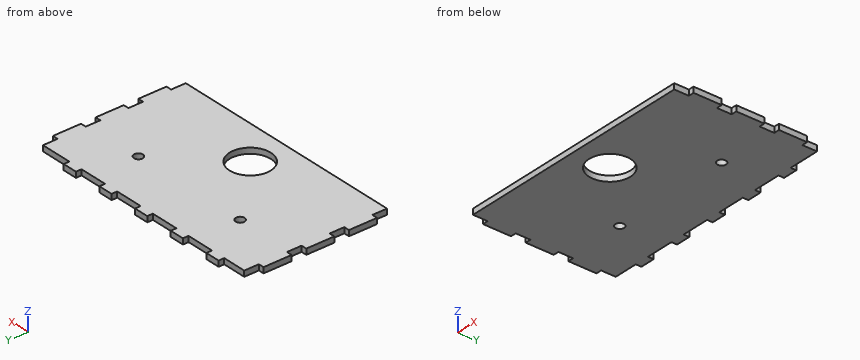
from build123d import *

# Parameters (mm, degrees)
SKETCH1_W               = 134.64
SKETCH1_H               = 76.2
BOSS_EXTRUDE1_DEPTH     = 3
SKETCH2_W               = 3
SKETCH2_H               = 7.8
CUT_EXTRUDE1_DEPTH      = 78.411836304
LPATTERN1_COUNT         = 4
LPATTERN1_PITCH         = 22.8
MIRROR4_COPY_1_SKETCH_W = 3
MIRROR4_COPY_1_SKETCH_H = 7.8
MIRROR4_COPY_1_DEPTH    = 78.411836304
MIRROR4_COPY_2_SKETCH_W = 3
MIRROR4_COPY_2_SKETCH_H = 7.8
MIRROR4_COPY_2_DEPTH    = 78.411836304
MIRROR4_COPY_3_SKETCH_W = 3
MIRROR4_COPY_3_SKETCH_H = 7.8
MIRROR4_COPY_3_DEPTH    = 78.411836304
SKETCH3_W               = 7.8
SKETCH3_H               = 3
BOSS_EXTRUDE2_DEPTH     = 3
LPATTERN2_COUNT         = 5
LPATTERN2_PITCH         = 22.8
SKETCH4_R               = 11
CUT_EXTRUDE2_DEPTH      = 79.931567829
SKETCH5_R               = 2.3749
CUT_EXTRUDE3_DEPTH      = 79.931567829


with BuildPart() as part:
    # Sketch1 → Boss-Extrude1 (new body)
    with BuildSketch(Plane.XY):
        Rectangle(SKETCH1_W, SKETCH1_H)
    extrude(amount=BOSS_EXTRUDE1_DEPTH)

    # Sketch2 → Cut-Extrude1 (cut, through all)
    with BuildSketch(Plane.XY.offset(3)):
        with Locations((-65.82, 34.2)):
            Rectangle(SKETCH2_W, SKETCH2_H)
    cut_extrude1 = extrude(amount=-CUT_EXTRUDE1_DEPTH, mode=Mode.SUBTRACT)

    # LPattern1: Cut-Extrude1 ×4
    with Locations(*[(0, -i * LPATTERN1_PITCH, 0) for i in range(1, LPATTERN1_COUNT)]):
        add(cut_extrude1, mode=Mode.SUBTRACT)

    # Mirror4: Cut-Extrude1 across plane
    add(cut_extrude1.mirror(Plane(origin=(0, 0, 0), x_dir=(0, 0, 1), z_dir=(1, 0, 0))), mode=Mode.SUBTRACT)

    # Mirror4 copy 1 sketch → Mirror4 copy 1 (cut, through all)
    with BuildSketch(Plane(origin=(0, -22.8, 3), x_dir=(-1, 0, 0), z_dir=(0, 0, 1))):
        with Locations((-65.82, -34.2)):
            Rectangle(MIRROR4_COPY_1_SKETCH_W, MIRROR4_COPY_1_SKETCH_H)
    extrude(amount=-MIRROR4_COPY_1_DEPTH, mode=Mode.SUBTRACT)

    # Mirror4 copy 2 sketch → Mirror4 copy 2 (cut, through all)
    with BuildSketch(Plane(origin=(0, -45.6, 3), x_dir=(-1, 0, 0), z_dir=(0, 0, 1))):
        with Locations((-65.82, -34.2)):
            Rectangle(MIRROR4_COPY_2_SKETCH_W, MIRROR4_COPY_2_SKETCH_H)
    extrude(amount=-MIRROR4_COPY_2_DEPTH, mode=Mode.SUBTRACT)

    # Mirror4 copy 3 sketch → Mirror4 copy 3 (cut, through all)
    with BuildSketch(Plane(origin=(0, -68.4, 3), x_dir=(-1, 0, 0), z_dir=(0, 0, 1))):
        with Locations((-65.82, -34.2)):
            Rectangle(MIRROR4_COPY_3_SKETCH_W, MIRROR4_COPY_3_SKETCH_H)
    extrude(amount=-MIRROR4_COPY_3_DEPTH, mode=Mode.SUBTRACT)

    # Sketch3 → Boss-Extrude2 (add)
    with BuildSketch(Plane(origin=(0, 38.1, 0), x_dir=(1, 0, 0), z_dir=(0, 1, 0))):
        with Locations((-47.62, -1.5)):
            Rectangle(SKETCH3_W, SKETCH3_H)
    boss_extrude2 = extrude(amount=BOSS_EXTRUDE2_DEPTH)

    # LPattern2: Boss-Extrude2 ×5
    with Locations(*[(i * LPATTERN2_PITCH, 0, 0) for i in range(1, LPATTERN2_COUNT)]):
        add(boss_extrude2)

    # Sketch4 → Cut-Extrude2 (cut, through all)
    with BuildSketch(Plane.XY.offset(3)):
        with Locations((0, -18.8)):
            Circle(SKETCH4_R)
    extrude(amount=-CUT_EXTRUDE2_DEPTH, mode=Mode.SUBTRACT)

    # Sketch5 → Cut-Extrude3 (cut, through all)
    with BuildSketch(Plane.XY.offset(3)):
        with Locations((32.526911935, 13.726911935)):
            Circle(SKETCH5_R)
        with Locations((-32.526911935, 13.726911935)):
            Circle(SKETCH5_R)
    extrude(amount=-CUT_EXTRUDE3_DEPTH, mode=Mode.SUBTRACT)


solid = part.part
Design review of the part built by this model. Coordinates are the model's own, in mm. Round coordinates to 2 decimals unless told otherwise and drop trailing zeros. Write each loop counter-clockwise with the first axis right and the second up, starting at its lowest first coordinate (ties: lowest second). Pieces come first, ordered by that corner, then holes. Notation, with made-up numbers: (-26, 18.25) - (-15, 18.25) arc R19 ccw to (-15, 41.25) - close; hole circle Ø9 at (-40, 29.5). An arc over 180 degrees is marked (long way). Return JSON: item names as keys, results as strings. Group by question number.
Item 1: Insertion check: P1, Ø1.5, axis at y = 39, z = 1, coming from the -X side; P2, Ø1, axis at x = 37.5, z = 2.5, coming from the +Y side; P3, Ø1.5, axis at y = 40, z = 1, coming from the +X side. Each pin has a flat end and moves straight along its axis. Give the tip position at first contact, or say it passes through.
Item 2: We need section A-A on y = -18.8. Write out the cut boundary in (x, z).
Item 3: We need section C-C on z = 0.6. Give the number of separate pieces and of enclosed holes in the cut face, and give its area (3 significant figures).
Item 4: We need section B-B on x = 0. Write out the cut boundary in (y, z).
Item 5: For probe 1 along X at (y, z) = (-18.5, 2.7); probe 2 along Y at (x, z) = (0, 1.35); probe 3 along Y at (x, z) = (-40, 0.25), list the stretches that pass through material, from the lowest coordinate up. Write a range as [from, to].
Model answer:
{
 "1": {"P1": "stops at x = -51.52", "P2": "stops at y = 38.1", "P3": "stops at x = 47.48"},
 "2": {"outline": "(-67.32, 0) - (-11, 0) - (-11, 3) - (-67.32, 3) - close; (11, 0) - (67.32, 0) - (67.32, 3) - (11, 3) - close"},
 "3": {"separate pieces": "1", "enclosed holes": "3", "area": "9,770 mm²"},
 "4": {"outline": "(-38.1, 0) - (-29.8, 0) - (-29.8, 3) - (-38.1, 3) - close; (-7.8, 0) - (41.1, 0) - (41.1, 3) - (-7.8, 3) - close"},
 "5": {"probe 1": "x = [-67.32, -11], [11, 67.32]", "probe 2": "y = [-38.1, -29.8], [-7.8, 41.1]", "probe 3": "y = [-38.1, 38.1]"}
}
